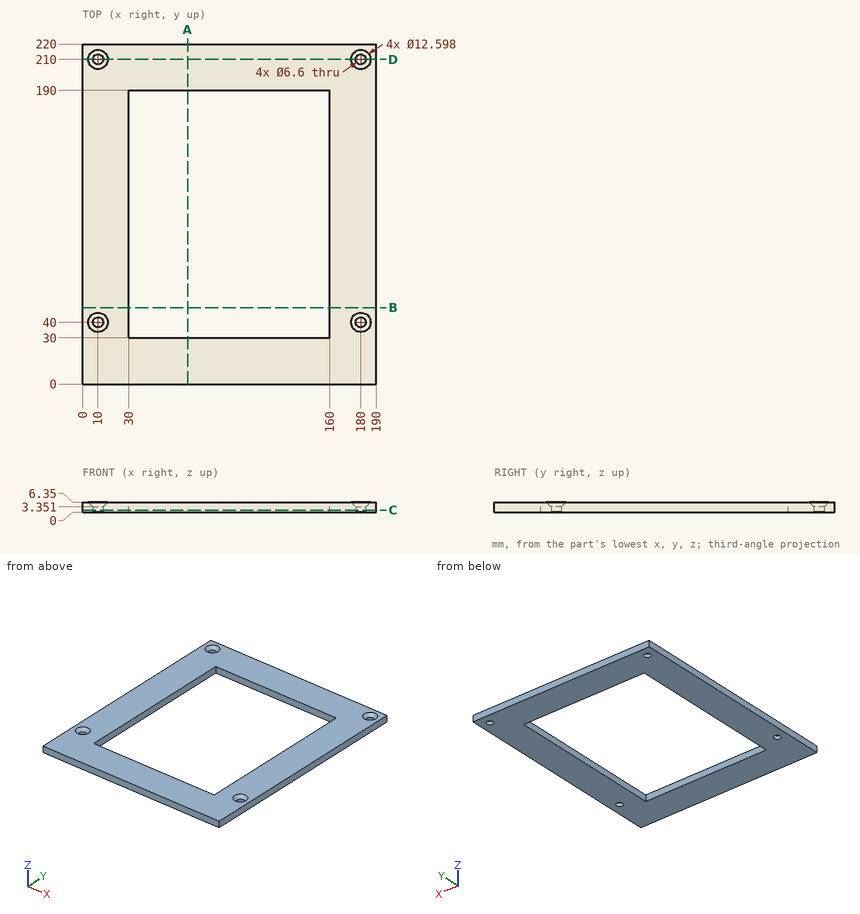
Input: dimensioned drawing with shaded views. Units: mm. Origin: part minimum x, y, z. Coordinates: 2 decimals unless noted, no trailing zeros. Order: outer loops, then holes, each group sorted by start corner. A loop starts at its lowest first (then second) coordinate and runs counter-clockwise, first axis right, second up.
(1) Section query D-D (y = 210). Return the cut outline in (x, z).
(2) Section query A-A (x = 68). Return the cut outline in (y, z), plus the area to 3 significant figures.
(3) Section query B-B (y = 49.5). Return the cut outline in (x, z), plus the area to 3 significant figures.
(4) Material intervals for probe 1 along X at (y, z) = (210, 1.95); probe 2 along Y at (x, z) = (10, 2.75); probe 3 along X at (y, z) = (40, 0.85), sorted ascending.
(5) First-contact query: pin 1 (6 mm diameter, centred on x = 180, y = 40, fed in from +Z); pin 2 (7.5 mm diameter, centred on x = 10, y = 40, fed in from +Z); pin 3 (8 mm diameter, centred on x = 97.5, y = 195.5, fed in from -Z). Flat tips, straight axial feed; report the tip coordinate or a pass-through.
(6) Section query C-C (z = 1.25). Return the cut outline in (x, y).
Solution:
1. outline: (0, 0) - (6.7, 0) - (6.7, 3.35) - (3.7, 6.35) - (0, 6.35) - close; (13.3, 0) - (176.7, 0) - (176.7, 3.35) - (173.7, 6.35) - (16.3, 6.35) - (13.3, 3.35) - close; (183.3, 0) - (190, 0) - (190, 6.35) - (186.3, 6.35) - (183.3, 3.35) - close
2. outline: (0, 0) - (30, 0) - (30, 6.35) - (0, 6.35) - close; (190, 0) - (220, 0) - (220, 6.35) - (190, 6.35) - close
2. area: 381 mm2
3. outline: (0, 0) - (30, 0) - (30, 6.35) - (0, 6.35) - close; (160, 0) - (190, 0) - (190, 6.35) - (160, 6.35) - close
3. area: 381 mm2
4. probe 1: x = 0 to 6.7, 13.3 to 176.7, 183.3 to 190
4. probe 2: y = 0 to 36.7, 43.3 to 206.7, 213.3 to 220
4. probe 3: x = 0 to 6.7, 13.3 to 30, 160 to 176.7, 183.3 to 190
5. pin 1: passes through
5. pin 2: stops at z = 3.8
5. pin 3: stops at z = 0
6. outline: (0, 0) - (190, 0) - (190, 220) - (0, 220) - close; hole circle Ø6.6 at (10, 40); hole circle Ø6.6 at (10, 210); hole (30, 30) - (160, 30) - (160, 190) - (30, 190) - close; hole circle Ø6.6 at (180, 40); hole circle Ø6.6 at (180, 210)
